```python
from build123d import *

# Parameters (mm, degrees)
SKETCH1_R           = 1
SKETCH1_R_2         = 3
BOSS_EXTRUDE1_DEPTH = 2
SKETCH2_R           = 0.5
CUT_EXTRUDE1_DEPTH  = 0.5


with BuildPart() as part:
    # Sketch1 → Boss-Extrude1 (new body)
    with BuildSketch(Plane.XY):
        with BuildLine():
            Line((-11.100190374, 3), (11.100190374, 3))
            ThreePointArc((11.100190374, 3), (13.067032348, 2.265288646), (14.070500235, 0.421021768))
            ThreePointArc((14.070500235, 0.421021768), (15.920210774, -10.795987627), (7.645834317, -3))
            Line((7.645834317, -3), (-7.645834317, -3))
            ThreePointArc((-7.645834317, -3), (-15.920210774, -10.795987627), (-14.070500235, 0.421021768))
            ThreePointArc((-14.070500235, 0.421021768), (-13.067032348, 2.265288646), (-11.100190374, 3))
        make_face()
        Circle(SKETCH1_R, mode=Mode.SUBTRACT)
        with Locations((-13.100190374, -5.5)):
            Circle(SKETCH1_R_2, mode=Mode.SUBTRACT)
        with Locations((13.100190374, -5.5)):
            Circle(SKETCH1_R_2, mode=Mode.SUBTRACT)
        with Locations((-11.100190374, 0)):
            Circle(SKETCH1_R, mode=Mode.SUBTRACT)
        with Locations((11.100190374, 0)):
            Circle(SKETCH1_R, mode=Mode.SUBTRACT)
    extrude(amount=BOSS_EXTRUDE1_DEPTH)

    # Sketch2 → Cut-Extrude1 (cut)
    with BuildSketch(Plane.XZ.offset(3)):
        with Locations((0, 1)):
            Circle(SKETCH2_R)
    extrude(amount=-CUT_EXTRUDE1_DEPTH, mode=Mode.SUBTRACT)


solid = part.part
```
Work out the finished part from the listing and answer in its coordinate system (mm). A direction names the side the tool comes from. Give positions to 0.01 mm unless a question says otherwise; leave off trailing zeros. Write each loop counter-clockwise with the first axis right and the second up, starting at its lowest first coordinate (ties: lowest second). Pieces come first, ordered by that corner, then holes.
(1) Straight lines are drawn through the part: line 1 (Y direction, x = 12, z = 0.9); line 2 (Z direction, x = 0, y = -2.9); line 3 (Y direction, x = 0, z = 1). For each, find the intervals that lie inside material, in ascending order.
Final values:
line 1: y = -11.4 to -8.29, -2.71 to -0.44, 0.44 to 2.86
line 2: z = 0 to 0.5, 1.5 to 2
line 3: y = -2.5 to -1, 1 to 3
(2) The part is cut by section D-D on y = 0. Write down the section's boundary in (x, z), plus the area to 3 significant figures.
Final values:
outline: (-15.5, 0) - (-12.1, 0) - (-12.1, 2) - (-15.5, 2) - close; (-10.1, 0) - (-1, 0) - (-1, 2) - (-10.1, 2) - close; (1, 0) - (10.1, 0) - (10.1, 2) - (1, 2) - close; (12.1, 0) - (15.5, 0) - (15.5, 2) - (12.1, 2) - close
area: 50.0 mm2
(3) The part is cut by section C-C on y = -5.5. Write down the section's boundary in (x, z), plus the area to 3 significant figures.
Final values:
outline: (-19.1, 0) - (-16.1, 0) - (-16.1, 2) - (-19.1, 2) - close; (-10.1, 0) - (-7.1, 0) - (-7.1, 2) - (-10.1, 2) - close; (7.1, 0) - (10.1, 0) - (10.1, 2) - (7.1, 2) - close; (16.1, 0) - (19.1, 0) - (19.1, 2) - (16.1, 2) - close
area: 24.0 mm2
(4) The part is cut by section B-B on z = 1. Write down the section's boundary in (x, y).
Final values:
outline: (-14.07, 0.42) arc R6 ccw (long way) to (-7.65, -3) - (-0.5, -3) - (-0.5, -2.5) - (0.5, -2.5) - (0.5, -3) - (7.65, -3) arc R6 ccw (long way) to (14.07, 0.42) arc R3 ccw to (11.1, 3) - (-11.1, 3) arc R3 ccw to start; hole circle Ø6 at (-13.1, -5.5); hole circle Ø2 at (-11.1, 0); hole circle Ø2 at (0, 0); hole circle Ø6 at (13.1, -5.5); hole circle Ø2 at (11.1, 0)
(5) The mould has two halves that part along Z. Classify faces 3 (the cylindrical face through (-0.108, -2.754, 0.512)), 4 (the cylindrical face through (-11.49, -2.97, 0.99)), 5 (the flat face through (0.3, -2.5, 2)): pulls with the +Z half, pulls with the -Z half, needs draft (parallel to the pull), parting line crosses it, or undercut.
Final values:
face 3: undercut
face 4: needs draft
face 5: pulls with the +Z half
(6) Which of the six approach directions +Z, -Z, +X, -X, +Y, -Y give full straight-line access (tool end or side, diameter ignored) to faces 1 (the flat face through (0, -2.5, 1)), 2 (the cylindrical face through (-13.09, 2.245, 0.986))?
Final values:
face 1: -Y
face 2: +Z, -Z, -X, +Y
(7) Flat-ended cylindrical pins translate along their axes: pin 1 Ø7 at (x, y) = (-13.1, -5.5) entering from -Z; pin 2 Ø1 at (x, z) = (-3.5, 1.5) entering from -Y; pin 3 Ø1.2 at (x, y) = (0, 0) entering from +Z. Find the tip coordinate at first contact, or state that the pin passes through.
Final values:
pin 1: stops at z = 0
pin 2: stops at y = -3
pin 3: passes through
(8) The part is cut by section A-A on x = 0. Write down the section's boundary in (y, z).
Final values:
outline: (-3, 0) - (-1, 0) - (-1, 2) - (-3, 2) - (-3, 1.5) - (-2.5, 1.5) - (-2.5, 0.5) - (-3, 0.5) - close; (1, 0) - (3, 0) - (3, 2) - (1, 2) - close
